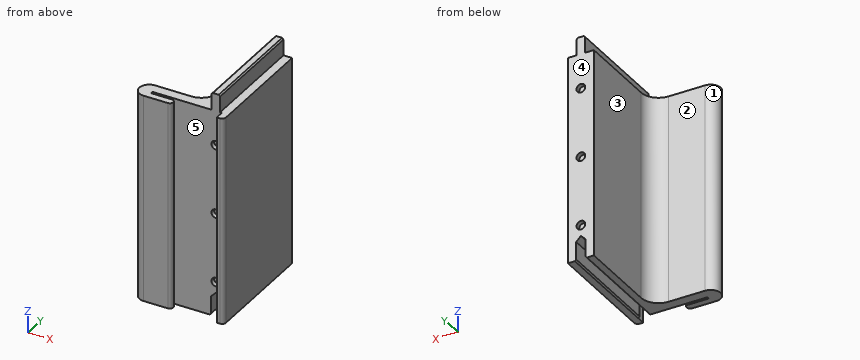
```python
from build123d import *

# Parameters (mm, degrees)
F1_DEPTH  = 76.2
F3_DEPTH  = 43.435
F4_W      = 3.175
F4_H      = 6.35
F5_DEPTH  = 40.005
F6_SIZE   = 0.508
F7_R      = 1.5875
F8_DEPTH  = 1.651
F9_R      = 1.5875
F10_DEPTH = 1.651


with BuildPart() as f1:
    # F0 (on Top) → F1 (new body)
    with BuildSketch(Plane.XY):
        with BuildLine():
            Line((2.54, 40.005), (-6.985, 40.005))
            Line((-6.985, 40.005), (-6.985, 10.16))
            ThreePointArc((-6.985, 10.16), (-8.8448719395, 5.6698719395), (-13.335, 3.81))
            Line((-13.335, 3.81), (-26.67, 3.81))
            ThreePointArc((-26.67, 3.81), (-30.2895, 0.1905), (-26.67, -3.429))
            Line((-26.67, -3.429), (-17.78, -3.429))
            ThreePointArc((-17.78, -3.429), (-16.51, -2.159), (-17.78, -0.889))
            Line((-17.78, -0.889), (-25.4, -0.889))
            Line((-25.4, -0.889), (-25.4, 0))
            Line((-25.4, 0), (0, 0))
            Line((0, 0), (0, -3.175))
            Line((0, -3.175), (1.2192, -3.175))
            ThreePointArc((1.2192, -3.175), (2.1531466366, -2.7881466366), (2.54, -1.8542))
            Line((2.54, -1.8542), (2.54, 40.005))
        make_face()
    extrude(amount=F1_DEPTH)

    # F2 (on face) → F3 (cut, through all)
    with BuildSketch(Plane(origin=(0, 40.005, 0), x_dir=(-1, 0, 0), z_dir=(0, 1, 0))):
        Polygon((0.508, 6.985), (0.508, 0), (3.937, 0), (3.937, 6.985), (2.2225, 8.6995), align=None)
    extrude(amount=-F3_DEPTH, mode=Mode.SUBTRACT)

    # F4 (on face) → F5 (join, through all)
    with BuildSketch(Plane(origin=(0, 40.005, 0), x_dir=(-1, 0, 0), z_dir=(0, 1, 0))):
        with Locations((2.2225, 79.375)):
            Rectangle(F4_W, F4_H)
    extrude(amount=-F5_DEPTH)

    # F6
    f6_edges = [f1.edges().sort_by_distance(p)[0] for p in [
        (-3.937, 20.0025, 0),
        (-0.508, 20.0025, 0),
        (-0.635, 20.0025, 82.55),
        (-3.81, 20.0025, 82.55),
    ]]
    chamfer(f6_edges, length=F6_SIZE)

    # F7 (on face) → F8 (cut)
    with BuildSketch(Plane(origin=(0, 40.005, 0), x_dir=(-1, 0, 0), z_dir=(0, 1, 0))):
        with Locations((2.2225, 12.7)):
            Circle(F7_R)
        with Locations((2.2225, 38.1)):
            Circle(F7_R)
        with Locations((2.2225, 63.5)):
            Circle(F7_R)
    extrude(amount=-F8_DEPTH, mode=Mode.SUBTRACT)

    # F9 (on face) → F10 (cut)
    with BuildSketch(Plane.XZ):
        with Locations((-2.2225, 12.7)):
            Circle(F9_R)
        with Locations((-2.2225, 38.1)):
            Circle(F9_R)
        with Locations((-2.2225, 63.5)):
            Circle(F9_R)
    extrude(amount=-F10_DEPTH, mode=Mode.SUBTRACT)


solid = f1.part
```
Geometry check sheet. Reference: the model listing, model coordinates, mm. Face numbers are marked on the shaded views. A direction names the side the tool comes from. Give positions to 0.01 mm unless a question says otherwise; leave off trailing zeros. Loops run counter-clockwise (first coordinate to the right, second up) from the corner with the lowest first, then second, coordinate; pieces in that order, holes last. Notation, with made-up numbers: (53, -27) - (69, -27) arc R19 cw to (69, -12) - close; hole circle Ø6 at (17, 68). An arc over 180 degrees is marked (long way). Use CSV: the item, a comma, the result in double quotes. Start each with the question number.
Q1. Access from +Z, -Z, +X, -X, +Y, -Y to the whole of each face (thin tool, end or side, straight path). Record for the marked faces 1 and 2.
Q2. Section check C-C, the plane x = -9. Record the cut outline in (y, z), and give its area (3 significant figures).
Q3. Go/stop test with flat-tipped pins: pin 1 Ø1 at (x, z) = (-2, 12) entering from +Y; pin 2 Ø14.5 at (x, z) = (-17, 53) entering from +Y; pin 3 Ø2.5 at (x, z) = (-23, 29.5) entering from +Y; pin 4 Ø2.5 at (x, z) = (-2.5, 63) entering from +Y (3 decimals). Record where each tip stops, or that it passes through.
Q4. Scan lines: probe 1 along X at (y, z) = (31, 4) (3 decimals); probe 2 along Y at (x, z) = (-20.5, 66); probe 3 along Y at (x, z) = (-0.5, 52) (3 decimals). Record each from-to range of solid material in increasing order. Write a range as from..to.
Q5. Release check for a two-part mould opening along X. For the marked faces 3, 4 and 5 record: +X half, -X half, draft (parallel to the pull), parting line (faces both ways), or undercut.
Findings below:
1,face 1,"+Z, -Z, -X"
1,face 2,"+Z, -Z, -X, +Y"
2,outline,"(0, 0) - (5.52, 0) - (5.52, 76.2) - (0, 76.2) - close"
2,area,"421 mm^2"
3,pin 1,"stops at y = 38.35"
3,pin 2,"stops at y = 4.92"
3,pin 3,"stops at y = 3.81"
3,pin 4,"stops at y = 40.005"
4,probe 1,"x = -6.985..-3.937, -0.508..2.54"
4,probe 2,"y = -3.43..-0.89, 0..3.81"
4,probe 3,"y = 0..40.005"
5,face 3,"-X half"
5,face 4,"draft"
5,face 5,"undercut"
